Read the model definition and answer for the solid it produces. Units are mm, in the model's axes. A direction names the side the tool comes from. Coordinates: 2 decimals unless noted, no trailing zeros. Write each loop counter-clockwise with the first axis right and the second up, starting at its lowest first coordinate (ties: lowest second). Pieces come first, ordered by that corner, then holes.
Item 1: A tool of negligible diameter and unlimited length cuts with its end or side. For faces 1 (the face through (-140, 0, -2)), 2 (the face through (-147.1, 13.7, -9.5)), 3 (the face through (-157.15, -41.99, -6.59)), 4 (the face through (-79, 29.5, -1)), from which of +Z, -Z, +X, -X, +Y, -Y can it reach the whole face along a straight path? Write none if from no direction.
Item 2: Section B-B (y = 0) is taken. Give the vertices of the cut face in (x, z), then the cut area to 3 significant figures.
Item 3: Determine the mould class of faces 5 (the face through (-157.15, 41.99, -6.59)), 6 (the face through (-95, 0, -3)), 7 (the face through (-63, 1, -13)) for opening direction Y: released by +Y, released by -Y, zero draft, split by the parting line, or undercut.
Item 4: Each of these flat-tipped pins is pushed along its axis until it touches: P1, Ø3.5, axis at x = -78.5, z = -1, coming from the +Y side; P2, Ø2.5, axis at x = -138.5, y = 0.5, coming from the +Z side; P3, Ø10, axis at x = -98.5, y = 26.5, coming from the +Z side; P4, Ø2, axis at x = -152, y = 37, coming from the +Z side. Where does it stop, or does it pass through?
Item 5: Section A-A (x = -129.25) is taken. Give the vertices of the cut face in (y, z).
Item 6: Straight lines are drawn through the part: probe 1 along Y at (x, z) = (-129.25, -6.25); probe 2 along X at (y, z) = (-22.5, -3.5); probe 3 along X at (y, z) = (3, -10). For each, find the intervals that lie inside material, in ascending order.
Item 7: Section D-D (x = -83.5) is taken. Give the vertices of the cut face in (y, z), then the cut area to 4 significant figures.
Item 8: Section C-C (y = 19.5) is taken. Give the vertices of the cut face in (x, z).
from build123d import *

# Parameters (mm, degrees)
SKETCH018_W         = 160
SKETCH018_H         = 90
PAD004_DEPTH        = 13
HOLE005_D           = 3.5
HOLE005_DEPTH       = 10
HOLE005_CBORE_D     = 4.2
HOLE005_CBORE_DEPTH = 5.2
HOLE005_TIPS_R      = 1.75
SKETCH020_R         = 8.5
POCKET008_DEPTH     = 13.001
SKETCH021_W         = 5
SKETCH021_H         = 12
SKETCH021_W_2       = 3.5
SKETCH021_H_2       = 57
SKETCH021_W_3       = 29
SKETCH021_H_3       = 10
POCKET009_DEPTH     = 5
SKETCH022_W         = 21.5
SKETCH022_H         = 46.5
SKETCH022_W_2       = 29
SKETCH022_H_2       = 57
SKETCH022_W_3       = 30
SKETCH022_H_3       = 12
POCKET010_DEPTH     = 1.5
SKETCH031_R         = 25.5
SKETCH031_R_2       = 22.5
POCKET016_DEPTH     = 7
PAD_DEPTH           = 5
FILLET_R            = 10
SKETCH034_W         = 29
SKETCH034_H         = 15.5
POCKET018_DEPTH     = 3
POCKET019_DEPTH     = 5
POCKET021_DEPTH     = 12


with BuildPart() as part:
    # Sketch018 → Pad004 (new body)
    with BuildSketch(Plane.XY):
        with Locations((-80, 0)):
            Rectangle(SKETCH018_W, SKETCH018_H)
    extrude(amount=-PAD004_DEPTH)

    # Hole005
    with Locations(Plane.XY):
        with Locations((-152, 37), (-8, 37), (-152, -37), (-8, -37)):
            CounterBoreHole(HOLE005_D / 2, HOLE005_CBORE_D / 2, HOLE005_CBORE_DEPTH, depth=HOLE005_DEPTH)

    # Hole005 tips → Hole005 tip 1 section 0
    with BuildSketch(Plane.XY.offset(-10), mode=Mode.PRIVATE) as hole005_tip_1_s0:
        with Locations((-152, 37)):
            Circle(HOLE005_TIPS_R)
    loft([hole005_tip_1_s0.sketch, Vertex(-152, 37, -11.051506)], mode=Mode.SUBTRACT)

    # Hole005 tips → Hole005 tip 2 section 0
    with BuildSketch(Plane.XY.offset(-10), mode=Mode.PRIVATE) as hole005_tip_2_s0:
        with Locations((-8, 37)):
            Circle(HOLE005_TIPS_R)
    loft([hole005_tip_2_s0.sketch, Vertex(-8, 37, -11.051506)], mode=Mode.SUBTRACT)

    # Hole005 tips → Hole005 tip 3 section 0
    with BuildSketch(Plane.XY.offset(-10), mode=Mode.PRIVATE) as hole005_tip_3_s0:
        with Locations((-152, -37)):
            Circle(HOLE005_TIPS_R)
    loft([hole005_tip_3_s0.sketch, Vertex(-152, -37, -11.051506)], mode=Mode.SUBTRACT)

    # Hole005 tips → Hole005 tip 4 section 0
    with BuildSketch(Plane.XY.offset(-10), mode=Mode.PRIVATE) as hole005_tip_4_s0:
        with Locations((-8, -37)):
            Circle(HOLE005_TIPS_R)
    loft([hole005_tip_4_s0.sketch, Vertex(-8, -37, -11.051506)], mode=Mode.SUBTRACT)

    # Sketch020 (on Face4 of Hole005) → Pocket008 (cut, through all)
    with BuildSketch(Plane.XY):
        with Locations((-129.25, 13)):
            Circle(SKETCH020_R)
        with Locations((-129.25, -13)):
            Circle(SKETCH020_R)
    extrude(amount=-POCKET008_DEPTH, mode=Mode.SUBTRACT)

    # Sketch021 (on Face4 of Pocket008) → Pocket009 (cut)
    with BuildSketch(Plane.XY):
        with Locations((-121, 0)):
            Rectangle(SKETCH021_W, SKETCH021_H)
        with Locations((-91.75, 0)):
            Rectangle(SKETCH021_W_2, SKETCH021_H_2)
        with Locations((-66.25, 0)):
            Rectangle(SKETCH021_W_2, SKETCH021_H_2)
        with Locations((-79, -33.5)):
            Rectangle(SKETCH021_W_3, SKETCH021_H_3)
    extrude(amount=-POCKET009_DEPTH, mode=Mode.SUBTRACT)

    # Sketch022 (on Face4 of Pocket009) → Pocket010 (cut)
    with BuildSketch(Plane.XY):
        with Locations((-129.25, 0)):
            Rectangle(SKETCH022_W, SKETCH022_H)
        with Locations((-79, 0)):
            Rectangle(SKETCH022_W_2, SKETCH022_H_2)
        with Locations((-108.5, 0)):
            Rectangle(SKETCH022_W_3, SKETCH022_H_3)
    extrude(amount=-POCKET010_DEPTH, mode=Mode.SUBTRACT)

    # Sketch031 (on Face7 of Pocket010) → Pocket016 (cut)
    with BuildSketch(Plane(origin=(0, 0, -13), x_dir=(1, 0, 0), z_dir=(0, 0, -1))):
        with Locations((-129.25, 0)):
            Circle(SKETCH031_R)
        with Locations((-129.25, 0)):
            Circle(SKETCH031_R_2, mode=Mode.SUBTRACT)
    extrude(amount=-POCKET016_DEPTH, mode=Mode.SUBTRACT)

    # Sketch033 (on Face8 of Pocket016) → Pad (join)
    with BuildSketch(Plane.XY.offset(-5)):
        Polygon((-87.9, -29), (-70.1, -29), (-70.1, -30), (-64.5, -30), (-64.5, -28.5), (-93.5, -28.5), (-93.5, -30), (-87.9, -30), align=None)
    extrude(amount=PAD_DEPTH)

    # Fillet
    fillet_edges = [part.edges().sort_by_distance(p)[0] for p in [
        (0, 45, -6.5),
        (0, -45, -6.5),
        (-160, -45, -6.5),
        (-160, 45, -6.5),
    ]]
    fillet(fillet_edges, radius=FILLET_R)

    # Sketch034 (on Face35 of Pad) → Pocket018 (cut)
    with BuildSketch(Plane.XY):
        with Locations((-79, 37.25)):
            Rectangle(SKETCH034_W, SKETCH034_H)
    extrude(amount=-POCKET018_DEPTH, mode=Mode.SUBTRACT)

    # Sketch035 (on Face48 of Pocket018) → Pocket019 (cut)
    with BuildSketch(Plane.XY.offset(-1.5)):
        with BuildLine():
            ThreePointArc((-134.8, 4.2), (-137.4, 6.8), (-140, 4.2))
            Line((-140, 4.2), (-140, -4.2))
            ThreePointArc((-140, -4.2), (-137.4, -6.8), (-134.8, -4.2))
            Line((-134.8, 4.2), (-134.8, -4.2))
        make_face()
    extrude(amount=-POCKET019_DEPTH, mode=Mode.SUBTRACT)

    # Sketch038 (on Face29 of Pocket019) → Pocket021 (cut)
    with BuildSketch(Plane.XZ.offset(-6)):
        with BuildLine():
            Line((-118.5, -5), (-118.5, -1.5))
            Line((-118.5, -1.5), (-93.5, -1.5))
            Line((-93.5, -1.5), (-96.414214, -4.414214))
            ThreePointArc((-97.828427, -5), (-97.06306, -4.847759), (-96.414214, -4.414214))
            Line((-118.5, -5), (-97.828427, -5))
        make_face()
    extrude(amount=POCKET021_DEPTH, mode=Mode.SUBTRACT)


solid = part.part
Established:
1. face 1: +Z
1. face 2: -Z
1. face 3: +Z, -Z, -X, -Y
1. face 4: +Z, +Y
2. outline: (-160, -13) - (-154.75, -13) - (-154.75, -6) - (-151.75, -6) - (-151.75, -13) - (-106.75, -13) - (-106.75, -6) - (-103.75, -6) - (-103.75, -13) - (0, -13) - (0, 0) - (-64.5, 0) - (-64.5, -5) - (-68, -5) - (-68, -1.5) - (-90, -1.5) - (-90, -5) - (-93.5, -5) - (-93.5, -1.5) - (-96.41, -4.41) arc R2 cw to (-97.83, -5) - (-123.5, -5) - (-123.5, -1.5) - (-134.8, -1.5) - (-134.8, -6.5) - (-140, -6.5) - (-140, 0) - (-160, 0) - close
2. area: 1,780 mm2
3. face 5: released by +Y
3. face 6: undercut
3. face 7: zero draft
4. P1: stops at y = 29.5
4. P2: stops at z = -6.5
4. P3: stops at z = 0
4. P4: stops at z = -10.45
5. outline: (-45, -13) - (-25.5, -13) - (-25.5, -6) - (-22.5, -6) - (-22.5, -13) - (-21.5, -13) - (-21.5, -1.5) - (-23.25, -1.5) - (-23.25, 0) - (-45, 0) - close; (-4.5, -13) - (4.5, -13) - (4.5, -1.5) - (-4.5, -1.5) - close; (21.5, -13) - (22.5, -13) - (22.5, -6) - (25.5, -6) - (25.5, -13) - (45, -13) - (45, 0) - (23.25, 0) - (23.25, -1.5) - (21.5, -1.5) - close
6. probe 1: y = -45 to -25.5, -22.5 to -21.5, -4.5 to 4.5, 21.5 to 22.5, 25.5 to 45
6. probe 2: x = -160 to -93.5, -90 to -68, -64.5 to 0
6. probe 3: x = -160 to -154.57, -151.55 to -106.95, -103.93 to 0
7. outline: (-45, -13) - (45, -13) - (45, -3) - (29.5, -3) - (29.5, 0) - (28.5, 0) - (28.5, -1.5) - (-28.5, -1.5) - (-28.5, 0) - (-29, 0) - (-29, -5) - (-38.5, -5) - (-38.5, 0) - (-45, 0) - close
7. area: 990.5 mm2
8. outline: (-160, -13) - (-145.68, -13) - (-145.68, -6) - (-140.47, -6) - (-140.47, -13) - (-134.73, -13) - (-134.73, -1.5) - (-140, -1.5) - (-140, 0) - (-160, 0) - close; (-123.77, -13) - (-118.03, -13) - (-118.03, -6) - (-112.82, -6) - (-112.82, -13) - (0, -13) - (0, 0) - (-64.5, 0) - (-64.5, -5) - (-68, -5) - (-68, -1.5) - (-90, -1.5) - (-90, -5) - (-93.5, -5) - (-93.5, 0) - (-118.5, 0) - (-118.5, -1.5) - (-123.77, -1.5) - close
